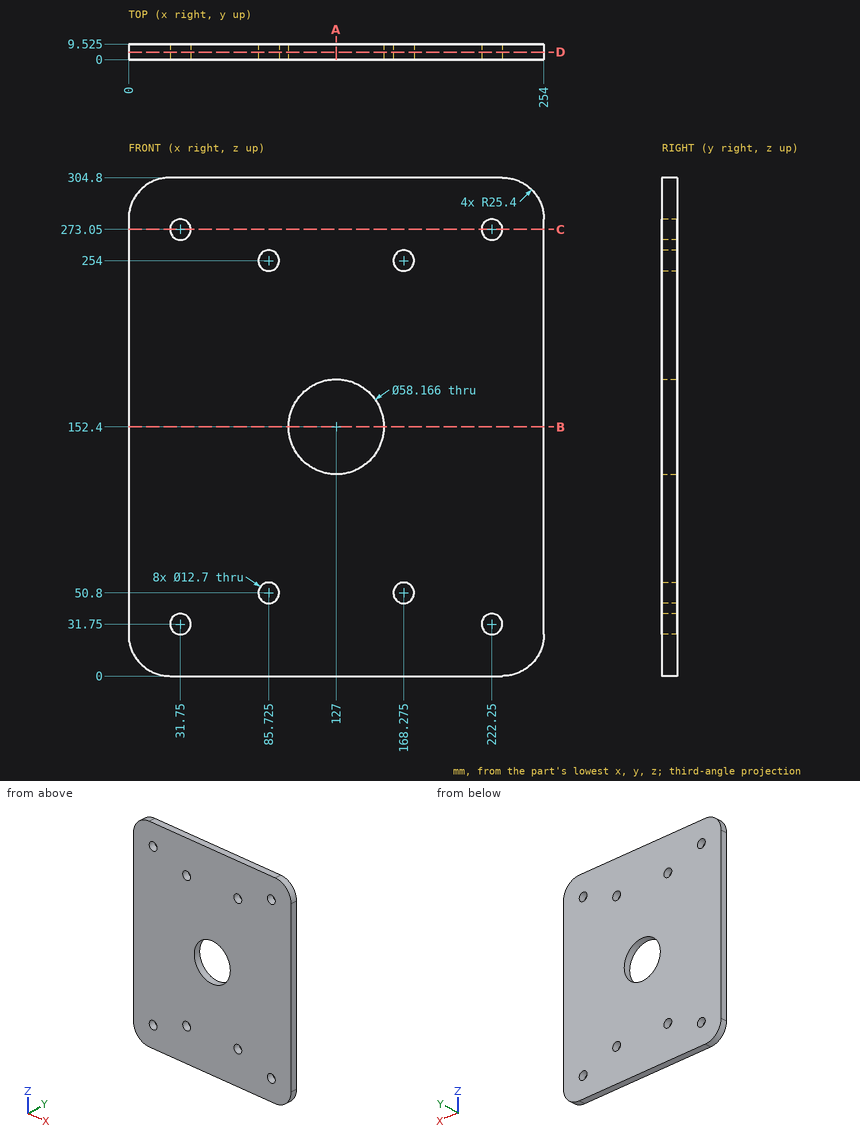
Can you work these out from the drawing? Everything is in mm from the part's minimum corner. Coordinates: 2 decimals unless noted, no trailing zeros. Loops run counter-clockwise (first coordinate to the right, second up) from the corner with the lowest first, then second, coordinate; pieces in that order, holes last.
1. Imagine slicing it at D-D, the plane y = 4.5. Count the separate pieces of the cut face and the enclosed holes in it, and give its area (3 significant figures).
2. For P1, Ø5, axis at x = 101, z = 149, coming from the -Y side, with a flat end and sliding along its axis, tell me the tip position at first contact or that it passes through.
3. Imagine slicing it at B-B, the plane z = 152.4. Please give me the cut outline in (x, y) (3 decimals), and give its area (3 significant figures).
4. Imagine slicing it at A-A, the plane x = 127. Please give me the cut outline in (y, z) (3 decimals).
5. I need wall thicknesses on L1, parallel to X at y = 1.25, z = 31; L2, parallel to X at y = 6.75, z = 254 (3 decimals); L3, parallel to Z at x = 31.75, y = 4.5. Which ranges of each line are inside material? Lowest first, please.
6. Imagine slicing it at C-C, the plane z = 273.05. Please give me the cut outline in (x, y) (3 decimals).
Taken from the geometry:
1. separate pieces: 1
1. enclosed holes: 9
1. area: 73,200 mm2
2. P1: passes through
3. outline: (0, 0) - (97.917, 0) - (97.917, 9.525) - (0, 9.525) - close; (156.083, 0) - (254, 0) - (254, 9.525) - (156.083, 9.525) - close
3. area: 1,870 mm2
4. outline: (0, 0) - (9.525, 0) - (9.525, 123.317) - (0, 123.317) - close; (0, 181.483) - (9.525, 181.483) - (9.525, 304.8) - (0, 304.8) - close
5. L1: x = 0 to 25.44, 38.06 to 215.94, 228.56 to 254
5. L2: x = 0 to 79.375, 92.075 to 161.925, 174.625 to 254
5. L3: z = 0 to 25.4, 38.1 to 266.7, 279.4 to 304.8
6. outline: (0, 0) - (25.4, 0) - (25.4, 9.525) - (0, 9.525) - close; (38.1, 0) - (215.9, 0) - (215.9, 9.525) - (38.1, 9.525) - close; (228.6, 0) - (254, 0) - (254, 9.525) - (228.6, 9.525) - close
